```python
from build123d import *

# Parameters (mm, degrees)
SKETCH1_W              = 29.21
SKETCH1_H              = 12.7
BOSS_EXTRUDE1_DEPTH    = 4.7625
F_10_32_TAPPED_HOLE1_D = 4.0386
F_10_CLEARANCE_HOLE1_D = 4.9784


with BuildPart() as part:
    # Sketch1 → Boss-Extrude1 (new, symmetric)
    with BuildSketch(Plane(origin=(0, 0, 0), x_dir=(0, 0, -1), z_dir=(1, 0, 0))):
        with Locations((-9.525, 0)):
            Rectangle(SKETCH1_W, SKETCH1_H)
    extrude(amount=BOSS_EXTRUDE1_DEPTH, both=True)

    # #10-32 Tapped Hole1 (through all)
    with Locations(Plane(origin=(0, 6.35, 0), x_dir=(1, 0, 0), z_dir=(0, 1, 0))):
        with Locations((0, 0)):
            Hole(F_10_32_TAPPED_HOLE1_D / 2)

    # #10 Clearance Hole1 (through all)
    with Locations(Plane(origin=(4.7625, 0, 0), x_dir=(0, 0, -1), z_dir=(1, 0, 0))):
        with Locations((-6.35, 0), (-19.05, 0)):
            Hole(F_10_CLEARANCE_HOLE1_D / 2)


solid = part.part
```
Check sheet for the modelled part. Datum: model origin and axes. Units: mm. Coordinates: 2 decimals unless noted, no trailing zeros. Order: outer loops, then holes, each group sorted by start corner. A loop starts at its lowest first (then second) coordinate and runs counter-clockwise, first axis right, second up. Notation, with made-up numbers: (31.25, -39) -> (82.25, -39) arc R13 cw to (82.25, -21) -> close; hole circle Ø7 at (-39.5, 52.5). An arc over 180 degrees is marked (long way). Write item = value, one per line. Start each with the question number.
1) Cross-section at A-A (x = 0). Enter the section's corners in (y, z), then the cut area to 3 significant figures.
2) Cross-section at C-C (y = 5.25). Enter the section's corners in (x, z).
3) Material ranges on L1, parallel to Y at x = 2, z = 6.35; L2, parallel to Z at x = 0, y = -0.25; L3, parallel to Z at x = 4, y = -0.75, recorded low to high.
4) Go/stop test with a flat-tipped pin: P1, Ø4, axis at y = 0, z = 6.35, coming from the -X side. Record where the tip stops, or that it passes through.
5) Cross-section at D-D (x = -3). Enter the section's corners in (y, z), then the cut area to 3 significant figures.
6) Mould release check, pull along X, two halves, no side actions. Record for faces 1 (the flat face through (4.762, 0, 10)), 2 (the flat face through (0, -6.35, 10)), 3 (the cylindrical face through (-1.926, -0.089, -0.607)): +X half, -X half, draft (parallel to the pull), parting line (faces both ways), or undercut.
7) Cross-section at B-B (z = 6.35). Enter the section's corners in (x, y), then the cut area to 3 significant figures.
Ans:
q1.outline = (-6.35, -5.08) -> (6.35, -5.08) -> (6.35, -2.02) -> (-6.35, -2.02) -> close; (-6.35, 2.02) -> (6.35, 2.02) -> (6.35, 24.13) -> (-6.35, 24.13) -> close; hole circle Ø4.98 at (0, 6.35); hole circle Ø4.98 at (0, 19.05)
q1.area = 281 mm²
q2.outline = (-4.76, -5.08) -> (4.76, -5.08) -> (4.76, 24.13) -> (-4.76, 24.13) -> close; hole circle Ø4.04 at (0, 0)
q3.L1 = -6.35 to -2.49, 2.49 to 6.35
q3.L2 = -5.08 to -2.02, 2.02 to 3.87, 8.83 to 16.57, 21.53 to 24.13
q3.L3 = -5.08 to 3.98, 8.72 to 16.68, 21.42 to 24.13
q4.P1 = through
q5.outline = (-6.35, -5.08) -> (6.35, -5.08) -> (6.35, 24.13) -> (-6.35, 24.13) -> close; hole circle Ø4.98 at (0, 6.35); hole circle Ø4.98 at (0, 19.05)
q5.area = 332 mm²
q6.face_1 = +X half
q6.face_2 = draft
q6.face_3 = undercut
q7.outline = (-4.76, -6.35) -> (4.76, -6.35) -> (4.76, -2.49) -> (-4.76, -2.49) -> close; (-4.76, 2.49) -> (4.76, 2.49) -> (4.76, 6.35) -> (-4.76, 6.35) -> close
q7.area = 73.5 mm²
